Autodesk Inventor part; units mm, degrees
ref_plane "YZ Plane" through (0, 0, 0) normal (1, 0, 0) x (0, 1, 0)
ref_plane "XZ Plane" through (0, 0, 0) normal (0, 1, 0) x (-1, 0, 0)
ref_plane "XY Plane" through (0, 0, 0) normal (0, 0, 1) x (1, 0, 0)
sketch "Esquisse1" plane through (0, 0, 0) normal (0, 1, 0) x (-1, 0, 0)
  arc A0 (-0.5, -2.4495) -> (0.5, -2.4495) centre (0, 0) ccw
  arc A1 (0.5, -3.4641) -> (-0.5, -3.4641) centre (0, 0) ccw
  arc A2 (0.5, -11.6834) -> (-0.5, -10.5279) centre (-4.5, -15) ccw
  arc A3 (0.5, -10.101) -> (-0.5, -9.2554) centre (-4.5, -15) ccw
  line L0 (-11.5, 3.5) -> (3.5, 3.5)
  line L1 (3.5, 3.5) -> (3.5, -17.5)
  line L2 (3.5, -17.5) -> (2.0383, -17.5)
  line L3 (-11.5, -17.5) -> (-11.5, 3.5)
  line L4 (-0.5, 0) -> (0.5, 0)
  line L5 (0.5, 0) -> (0.5, -2.4495)
  line L6 (0.5, -15) -> (-0.5, -15)
  line L7 (-0.5, -15) -> (-0.5, -10.5279)
  line L8 (0.5, -10.101) -> (0.5, -15)
  line L9 (-0.5, -9.2554) -> (-0.5, -3.4641)
  arc A4 (2.0383, -17.5) -> (0.5, -10.101) centre (-4.5, -15) ccw
  arc A5 (0.9544, -17.5) -> (0.5, -11.6834) centre (-4.5, -15) ccw
  line L10 (2.0383, -17.5) -> (0.9544, -17.5)
  line L11 (0.9544, -17.5) -> (-11.5, -17.5)
  arc A6 (-0.5, -10.5279) -> (0.9544, -17.5) centre (-4.5, -15) ccw
  arc A7 (-0.5, -9.2554) -> (2.0383, -17.5) centre (-4.5, -15) ccw
  line L12 (-0.5, -10.5279) -> (-0.5, -9.2554)
  arc A8 (0.5, -2.4495) -> (-0.5, -2.4495) centre (0, 0) ccw
  arc A9 (-0.5, -3.4641) -> (0.5, -3.4641) centre (0, 0) ccw
  line L13 (-0.5, -3.4641) -> (-0.5, -2.4495)
  line L14 (0.5, -2.4495) -> (0.5, -3.4641)
  line L15 (0.5, -3.4641) -> (0.5, -10.101)
  line L16 (-0.5, -2.4495) -> (-0.5, 0)
  dimension "d0" = 5
  dimension "d1" = 1
  dimension "d2" = 14
  dimension "d3" = 1
  dimension "d4" = 15
  dimension "d6" = 8
  dimension "d7" = 21
  dimension "d9" = 1
  dimension "d10" = 0.5
extrude "Extrusion1" add sketch "Esquisse1" against normal blind 9 contours L13 A1 L14 A8 | A9 L15 A3 L9 | A3 L8 A2 L12 | A4 L10 A5 L8
sketch "Esquisse2" plane through (0, 0, 0) normal (0, 1, 0) x (1, 0, 0)
  line L0 (0.5, 3.4641) -> (0.5, 2.4495)
  arc A0 (-0.5, 2.4495) -> (0.5, 2.4495) centre (0, 0) ccw
  line L1 (-0.5, 2.4495) -> (-0.5, 3.4641)
  arc A1 (-0.5, 2.4495) -> (0.5, 2.4495) centre (0, 0) ccw
  arc A2 (-0.5, 3.4641) -> (0.5, 3.4641) centre (0, 0) ccw
  arc A3 (0.5, 2.4495) -> (-0.5, 2.4495) centre (0, 0) ccw
  arc A4 (0.5, 3.4641) -> (-0.5, 3.4641) centre (0, 0) ccw
extrude "Extrusion2" add sketch "Esquisse2" against normal blind 9 contours L0 A3 L1 A4
sketch "Esquisse3" plane through (0, 0, 0) normal (0, 1, 0) x (1, 0, 0)
  circle A0 centre (0, 0) radius 2.5
  arc A1 (-0.9544, 17.5) -> (0.5, 10.5279) centre (4.5, 15) ccw
  line L0 (-0.9544, 17.5) -> (-2.0383, 17.5)
  arc A2 (-0.5, 3.4641) -> (0.5, 3.4641) centre (0, 0) ccw
  line L1 (5.5, 17.5) -> (-4.5, 17.5)
  line L2 (-4.5, 17.5) -> (-4.5, 12)
  line L3 (-4.5, 12) -> (5.5, 12)
  line L4 (5.5, 12) -> (5.5, 17.5)
  arc A3 (3.5, 2.8284) -> (-4.5, 0) centre (0, 0) ccw
  line L5 (-4.5, 0) -> (-2.5, 0)
  line L6 (3.5, 0) -> (3.5, 2.8284)
  line L7 (3.5, 12) -> (-4.5, 12)
  line L8 (-4.5, 12) -> (-4.5, 0)
  line L9 (5.5, 12) -> (3.5, 10)
  line L10 (3.5, 2.8284) -> (3.5, 12)
  arc A4 (-4.5, 0) -> (3.5, 2.8284) centre (0, 0) ccw
  arc A5 (2.5, 0) -> (-2.5, 0) centre (0, 0) ccw
  line L11 (2.5, 0) -> (3.5, 0)
  line L12 (-2.5, 0) -> (2.5, 0)
  arc A6 (-2.5, 0) -> (2.5, 0) centre (0, 0) ccw
  dimension "d15" = 1
  dimension "d16" = 3
  dimension "d18" = 1
  dimension "d19" = 8
  dimension "d20" = 135
extrude "Extrusion3" add sketch "Esquisse3" along normal blind 1 contours L11 A2 L5 A0 | A0 L5 A3 L6 L11 | L6 A4 L5 A2 | A3 L8 L3 L10 | L10 L3 L9 | L2 L1 L0 A1 L3 | L3 A1 L1 L4
sketch "Esquisse4" plane through (0, -9, 0) normal (0, -1, 0) x (1, 0, 0)
  arc A0 (0.5, -3.4641) -> (-0.5, -3.4641) centre (0, 0) ccw
  line L0 (-0.5, -3.4641) -> (-0.5, -10.101)
  line L1 (-2.0383, -17.5) -> (-0.9544, -17.5)
  line L2 (0.5, -10.5279) -> (0.5, -3.4641)
  circle A1 centre (0, 0) radius 2.5
  line L3 (-3.5, 0) -> (-2.5, 0)
  line L4 (3.5, 0) -> (3.5, -10)
  line L5 (3.5, -17.5) -> (-3.5, -17.5)
  line L6 (-3.5, -17.5) -> (-3.5, 0)
  arc A2 (3.5, 0) -> (-3.5, 0) centre (0, 0) ccw
  arc A3 (-2.5, 0) -> (2.5, 0) centre (0, 0) ccw
  line L7 (3.5, -17.5) -> (5.5, -17.5)
  line L8 (5.5, -17.5) -> (5.5, -12)
  line L9 (5.5, -12) -> (3.5, -12)
  line L10 (3.5, -12) -> (3.5, -17.5)
  line L11 (5.5, -12) -> (3.5, -12)
  line L12 (3.5, -12) -> (3.5, -10)
  line L13 (3.5, -10) -> (5.5, -10)
  line L14 (5.5, -10) -> (5.5, -12)
  arc A4 (0.5, -3.4641) -> (3.5, 0) centre (0, 0) ccw
  arc A5 (-0.5, -3.4641) -> (0.5, -3.4641) centre (0, 0) ccw
  arc A6 (-3.5, 0) -> (-0.5, -3.4641) centre (0, 0) ccw
  arc A7 (2.5, 0) -> (-2.5, 0) centre (0, 0) ccw
  line L15 (2.5, 0) -> (3.5, 0)
  line L16 (-2.5, 0) -> (2.5, 0)
  line L17 (3.5, -10) -> (3.5, -12)
  line L18 (3.5, -12) -> (3.5, -17.5)
  line L19 (3.5, -10) -> (5.5, -12)
extrude "Extrusion4" add sketch "Esquisse4" along normal blind 1 contours A5 A0 L3 A1 L15 | A0 L4 L12 L10 L5 L1 L6 A5 | L15 A1 L3 A0 | L9 L8 L7 L10
sketch "Esquisse5" plane through (0, 0, 0) normal (0, -1, 0) x (1, 0, 0)
  arc A0 (-0.5, -10.101) -> (-2.0383, -17.5) centre (4.5, -15) ccw
  circle A1 centre (4.5, -15) radius 0.5
  dimension "d25" = 1
extrude "Extrusion5" cut sketch "Esquisse5" along normal through all both and the other way through all
properties part number "tendeur"
The listing builds one solid part. Answer for the finished solid, in the listing's coordinates (mm). A direction names the side the tool comes from. Round coordinates to 2 decimals unless told otherwise and drop trailing zeros. Loops run counter-clockwise (first coordinate to the right, second up) from the corner with the lowest first, then second, coordinate; pieces in that order, holes last. Notation, with made-up numbers: (-7.75, -23) - (6.25, -23) arc R8 cw to (6.25, -9) - close; hole circle Ø4 at (85, 56). An arc over 180 degrees is marked (long way). Return JSON: item names as keys, results as strings. Group by question number.
1. Each of these flat-tipped pins is pushed along its axis until it touches: P1, Ø3, axis at x = 3, y = -4.5, coming from the -Z side; P2, Ø1, axis at y = -3, z = -11.5, coming from the -X side; P3, Ø1.1, axis at x = 5, y = -9.5, coming from the +Z side; P4, Ø3, axis at x = 0, z = 0, coming from the +Y side. Where does it stop, or does it pass through?
2. Consider probe 1 along Y at (x, z) = (1, -6.5); probe 2 along Z at (x, y) = (4.5, -9.35); probe 3 along X at (y, z) = (-9.5, -15). Determine where each line is inside the solid, lowest interval first.
3. Which of the six approach directions +Z, -Z, +X, -X, +Y, -Y give full straight-line access (tool end or side, diameter ignored) to faces 4 (the cylindrical face through (-2.365, -4.437, -13.63)), 5 (the flat face through (0.5, -4, -7)), 6 (the flat face through (-3.5, -9.5, -8.9))?
4. The mould has two halves that part along Y. Classify faces 1 (the flat face through (-4.5, 0.5, -8.9)), 2 (the flat face through (0, -10, -9)), 3 (the flat face through (-2, -9, -9)): pulls with the +Y half, pulls with the -Y half, needs draft (parallel to the pull), parting line crosses it, or undercut.
5. The part is cut by section B-B on x = 0. Determine the outline of the cut face in (y, z), then the cut area to 3 significant figures.
6. The part is cut by section A-A on z = -15. Determine the outline of the cut face in (x, y), then the cut area to 3 significant figures.
7. The part is cut by section C-C on y = -1. Determine the outline of the cut face in (x, z).
8. The part is cut by section D-D on x = 3.75. Determine the outline of the cut face in (y, z), then the cut area to 3 significant figures.
Resolved:
{
 "1": {"P1": "stops at z = -3.16", "P2": "stops at x = -1.82", "P3": "stops at z = -12", "P4": "passes through"},
 "2": {"probe 1": "y = -10 to -9, 0 to 1", "probe 2": "z = -17.5 to -15.5, -14.5 to -12", "probe 3": "x = -3.5 to 4, 5 to 5.5"},
 "3": {"face 4": "-X", "face 5": "-Z, +X", "face 6": "+Z, -Z, -X, -Y"},
 "4": {"face 1": "needs draft", "face 2": "pulls with the -Y half", "face 3": "undercut"},
 "5": {"outline": "(-10, -17.5) - (-9, -17.5) - (-9, -11.03) - (0, -11.03) - (0, -17.5) - (1, -17.5) - (1, -2.5) - (-9, -2.5) - (-10, -2.5) - close; (-10, 2.5) - (0, 2.5) - (1, 2.5) - (1, 4.5) - (0, 4.5) - (0, 3.5) - (-10, 3.5) - close", "area": "119 mm²"},
 "6": {"outline": "(-4.5, 0) - (-2.5, 0) - (-2.5, -9) - (-3.5, -9) - (-3.5, -10) - (4, -10) - (4, -9) - (-1.5, -9) - (-1.5, 0) - (4, 0) - (4, 1) - (-4.5, 1) - close; (5, -10) - (5.5, -10) - (5.5, -9) - (5, -9) - close; (5, 0) - (5.5, 0) - (5.5, 1) - (5, 1) - close", "area": "26.0 mm²"},
 "7": {"outline": "(-2.04, -17.5) - (-0.95, -17.5) arc R6 cw to (-0.5, -11.68) arc R6 cw to (0.5, -10.53) - (0.5, -3.46) arc R3.5 ccw (long way) to (-0.5, -3.46) - (-0.5, -10.1) arc R7 ccw to start; hole circle Ø5 at (0, 0)"},
 "8": {"outline": "(-10, -17.5) - (-9, -17.5) - (-9, -12) - (-10, -12) - close; (0, -17.5) - (1, -17.5) - (1, -10.25) - (0, -10.25) - close; (0, -2.49) - (1, -2.49) - (1, 2.49) - (0, 2.49) - close", "area": "17.7 mm²"}
}
